```python
from build123d import *

# Parameters (mm, degrees)
F2_R = 17.75
F0_R = 12.5
F4_T = -3
F7_D = 3


with BuildPart() as f3:
    # F2 (on offset) → F3 section 0
    with BuildSketch(Plane.XZ.offset(25)):
        Circle(F2_R)
    # F0 (on Front) → F3 section 1
    with BuildSketch(Plane.XZ):
        Circle(F0_R)
    loft()

    # F4
    f4_openings = [f3.faces().sort_by_distance(p)[0] for p in [
        (0, -25, 0),
    ]]
    offset(amount=F4_T, openings=f4_openings, kind=Kind.INTERSECTION)

    # F7 (through all)
    with Locations(Plane(origin=(0, 0, 0), x_dir=(-1, 0, 0), z_dir=(0, 1, 0))):
        with Locations((0, 0)):
            Hole(F7_D / 2)


solid = f3.part
```
Design review of the part built by this model. Coordinates are the model's own, in mm. A direction names the side the tool comes from. Give positions to 0.01 mm unless a question says otherwise; leave off trailing zeros. Loops run counter-clockwise (first coordinate to the right, second up) from the corner with the lowest first, then second, coordinate; pieces in that order, holes last. Notation, with made-up numbers: (46, -16.5) -> (72, -16.5) arc R17 cw to (72, -8.5) -> close; hole circle Ø1 at (79, -23). An arc over 180 degrees is marked (long way). Write each question's results on one line, items separated by ' | '.
Q1. For pin 1 Ø6 at (x, y) = (1.5, -8.5) entering from -Z; pin 2 Ø1.5 at (y, z) = (-21.5, 12) entering from +X; pin 3 Ø1.5 at (y, z) = (-10, 10) entering from +X, all flat-tipped, find the tip position at first contact; note any pin that passes through.
Reply:
pin 1: stops at z = -14.88 | pin 2: stops at x = 12.8 | pin 3: stops at x = 11.33
Q2. The part is to be moulded in two halves that separate along X. For faces 1 (the face through (3, -25, 15)), 2 (the face through (-1.5, -1.52, 0.07)), 3 (the face through (-3.14, -9.55, -14.16)), 4 (the face through (-9.387, -11.402, -7.198)), say which applies: +X half, -X half, draft (parallel to the pull), parting line (faces both ways), or undercut.
Reply:
face 1: draft | face 2: undercut | face 3: parting line | face 4: undercut
Q3. Take a section at C-C, the plane y = -15. Write out the cut boundary in (x, z), plus the area to 3 significant figures.
Reply:
outline: circle Ø31.3 at (0, 0); hole circle Ø25.17 at (0, 0) | area: 272 mm²
Q4. Machinability: for faces 5 (the face through (0, -3, -2)), 6 (the face through (0, 0, -3)), which of the approach directions +Z, -Z, +X, -X, +Y, -Y give a long, thin tool a straight path to every point of the face, cutting with its end or side? Answer none if there is none.
Reply:
face 5: -Y | face 6: +Z, -Z, +X, -X, +Y
Q5. Take a section at B-B, the plane y = -2.5. Write out the cut boundary in (x, z) (3 decimals), plus the area to 3 significant figures.
Reply:
outline: circle Ø26.05 at (0, 0); hole circle Ø3 at (0, 0) | area: 526 mm²
Q6. Take a section at A-A, the plane x = 0. Write out the cut boundary in (y, z), plus the area to 3 significant figures.
Reply:
outline: (-25, -17.75) -> (0, -12.5) -> (0, -1.5) -> (-3, -1.5) -> (-3, -10.06) -> (-25, -14.68) -> close; (-25, 14.68) -> (-3, 10.06) -> (-3, 1.5) -> (0, 1.5) -> (0, 12.5) -> (-25, 17.75) -> close | area: 203 mm²
Q7. Wall thickness on L1, parallel to Y at x = 9, z = -3; L2, parallel to Z at x = -5, y = -11; L3, parallel to Z at x = 0, y = -1.35: over which ranges is each line inside the solid? List them lowest first.
Reply:
L1: y = -3 to 0 | L2: z = -13.94 to -10.63, 10.63 to 13.94 | L3: z = -12.78 to -1.5, 1.5 to 12.78
